Answer from the drawing. Dimensions are ordinates in mm from the lowest x, y and z of the part. Round coordinates to 2 decimals unless told otherwise and drop trailing zeros. Order: outer loops, then holes, each group sorted by start corner. A loop starts at its lowest first (then second) coordinate and runs counter-clockwise, first axis right, second up. Notation, with made-up numbers: M 84,40.5 L 89,40.5 A18 cw 89,57.5 Z; hole C -12.75,35.25 d9. An arc over 180 degrees is marked long. Use one line per item in the form item = value. Start each with the question number.
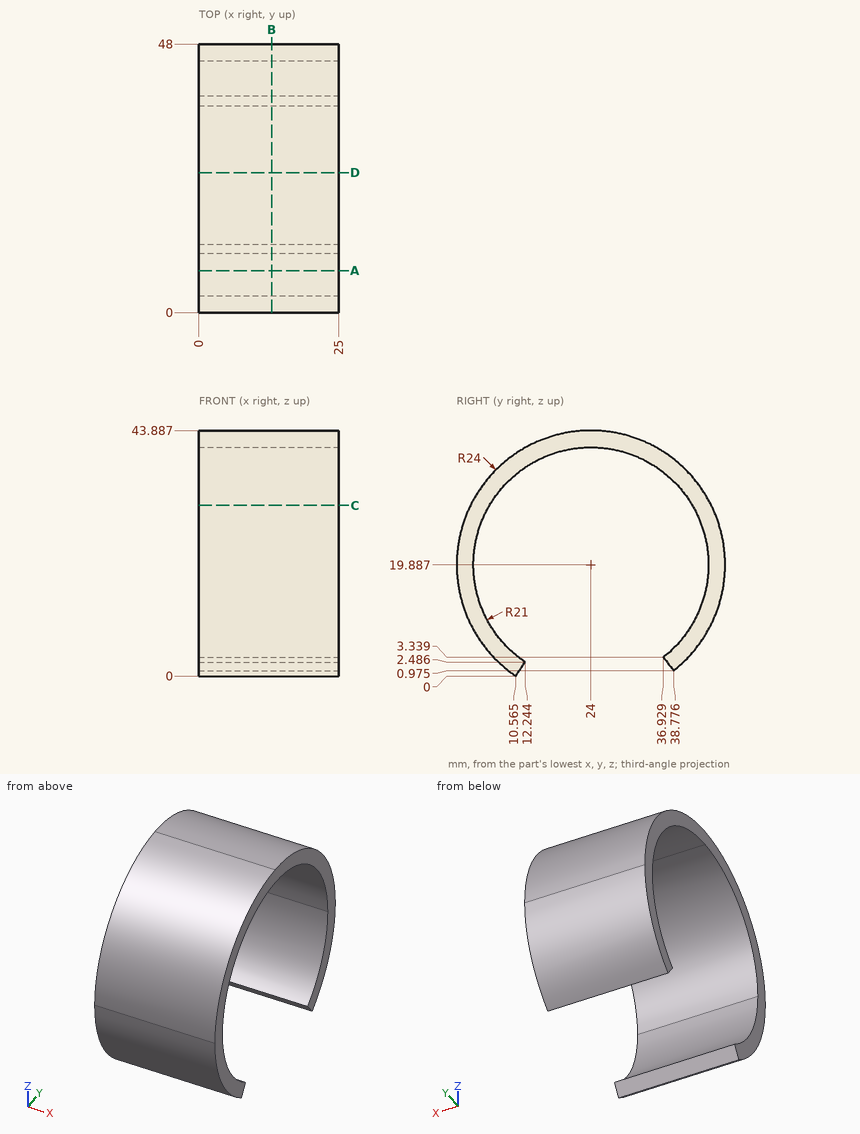
Item 1: Find the intervals of material crossed by L1, parallel to Z at x = 13.75, y = 40 (1 decimal); L2, parallel to Z at x = 4.25, y = 10 (1 decimal); L3, parallel to Y at x = 19.5, z = 8.5 (1 decimal), in increasing order. Write a range as [from, to].
Item 2: Section B-B (x = 13) is taken. Write down the section's boundary in (y, z) (1 decimal).
Item 3: Section A-A (y = 7.5) is taken. Write down the section's boundary in (x, z), and give its area (3 significant figures).
Item 4: Section D-D (y = 25) is taken. Write down the section's boundary in (x, z).
Item 5: Given P1, Ø2, axis at x = 20, z = 20.5, coming from the +Y side; P2, Ø6, axis at x = 4, y = 29.5, coming from the +Z side; P3, Ø3, axis at x = 9.5, y = 6, coming from the -Z side; P4, Ø10, axis at x = 9, y = 15.5, coming from the -Z side, each flat-ended and moving along its own axis, determine where each tip first touches the part or whether it passes through.
Item 6: Section C-C (z = 30.5) is taken. Write down the section's boundary in (x, y), and give its area (3 significant figures).
The answers:
q1.L1 = [2, 6.3], [33.5, 37.8]
q1.L2 = [0.4, 4.2], [35.5, 39.4]
q1.L3 = [2.9, 6.4], [41.6, 45.1]
q2.outline = M 0,19.9 A24 ccw 10.6,0 L 12.2,2.5 A21 cw 3,19.9 A21 cw 24,40.9 A21 cw 45,19.9 A21 cw 36.9,3.3 L 38.8,1 A24 ccw 48,19.9 A24 ccw 24,43.9 A24 ccw Z
q3.outline = M 0,2.46 L 25,2.46 L 25,6.9 L 0,6.9 Z; M 0,32.88 L 25,32.88 L 25,37.32 L 0,37.32 Z
q3.area = 222 mm²
q4.outline = M 0,40.86 L 25,40.86 L 25,43.87 L 0,43.87 Z
q5.P1 = 48
q5.P2 = 43.76
q5.P3 = 2.46
q5.P4 = 0
q6.outline = M 0,2.47 L 25,2.47 L 25,5.88 L 0,5.88 Z; M 0,42.12 L 25,42.12 L 25,45.53 L 0,45.53 Z
q6.area = 170 mm²
